Source: CAD feature listing. Evaluate the final solid. Frame: model axes, mm. Face numbers are marked on the shaded views. A direction names the side the tool comes from. Give positions to 0.01 mm unless a question says otherwise; leave off trailing zeros. Write each loop counter-clockwise with the first axis right and the second up, starting at its lowest first coordinate (ties: lowest second). Pieces come first, ordered by that corner, then holes. Notation, with made-up numbers: (-0.75, 52.25) -> (24.25, 52.25) arc R14 ccw to (24.25, 77.25) -> close; hole circle Ø9 at (63.5, -33). An arc over 180 degrees is marked (long way). Answer as a JSON object with one key per item and string values. Group by question number.
Item 1: Section query B-B on y = 16. Return the cut outline in (x, z) (1 decimal), plus the area to 3 significant figures.
Item 2: Section query A-A on z = -2125.5. Return the cut outline in (x, y), plus the area to 3 significant figures.
Item 3: Section query C-C on x = -18.5. Return the cut outline in (y, z), plus the area to 3 significant figures.
Item 4: Section query D-D on y = 61. Return the cut outline in (x, z), plus the area to 3 significant figures.
Item 5: Access query for the marked faces 4 and 5. Directions: +Z, -Z, +X, -X, +Y, -Y. A direction counts if a zero-diameter tool reaches every point of the face in a straight line with its end or side. Return the directions, or none.
Item 6: Pull-direction query (X, two-part tool) for the marked faces 1, 2 and 3; classes: pulls with the +X half, pulls with the -X half, needs draft (parallel to the pull), parting line crosses it, or undercut.
Item 7: Ray query, probe 1 along X at (y, z) = (5, -2128); probe 2 along Z at (x, y) = (28.5, 9); probe 3 along X at (y, z) = (24, -2125.25). Return the intervals inside material, ascending. Write a range as from..to.
Item 8: First-contact query: pin 1 Ø4.5 at (x, z) = (-39, -2123.5) entering from -Y; pin 2 Ø1.7 at (x, z) = (-25.5, -2116) entering from +Y; pin 3 Ø1.7 at (y, z) = (-16, -2116) entering from +X; pin 4 Ø8 at (y, z) = (61, -2123) entering from -X. Flat tips, straight axial feed; report the tip coordinate or a pass-through.
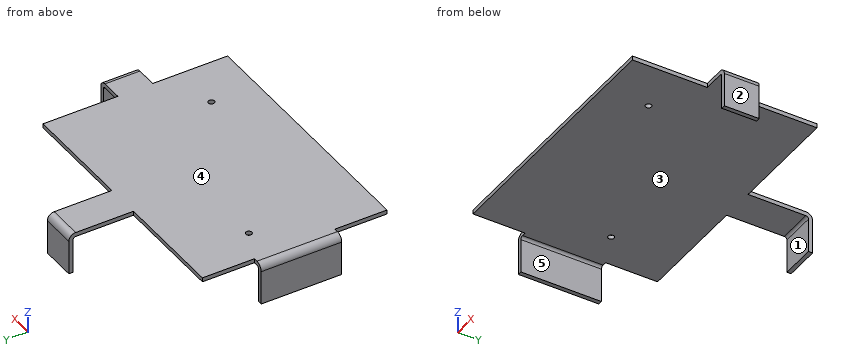
from build123d import *

# Parameters (mm, degrees)
BASE_FLANGE1_DEPTH             = 1.5875
EDGE_FLANGE1_STRIP_W           = 8.35
EDGE_FLANGE1_STRIP_H           = 1.5875
EDGE_FLANGE1_STRIP_CUT_DEPTH   = 30.48
EDGE_FLANGE1_STRIP_2_W         = 8.35
EDGE_FLANGE1_STRIP_2_H         = 1.5875
EDGE_FLANGE1_STRIP_CUT_2_DEPTH = 13.208
EDGE_FLANGE1_STRIP_3_W         = 8.35
EDGE_FLANGE1_STRIP_3_H         = 1.5875
EDGE_FLANGE1_STRIP_CUT_3_DEPTH = 13.208
EDGE_FLANGE1_DEPTH             = 30.48
EDGE_FLANGE1_BEND_DEPTH        = 13.208
EDGE_FLANGE1_BEND_2_DEPTH      = 13.208
F_4_40_TAPPED_HOLE2_D          = 2.2606
F_4_40_TAPPED_HOLE2_DEPTH      = 7.62
F_4_40_TAPPED_HOLE2_TIP        = 0.679152758


# Sheet-metal steps are written as plain solids
with BuildPart() as part:
    # Sketch4 → Base-Flange1 (new body)
    with BuildSketch(Plane.XY.offset(-2116.63312276)):
        Polygon((69.238438529, 17.87770801), (69.238438529, 4.66970801), (60.348438529, 4.66970801), (60.348438529, -23.65129199), (-37.441561471, -23.65129199), (-37.441561471, -3.96629199), (-39.981561471, -3.96629199), (-39.981561471, 26.51370801), (-37.441561471, 26.51370801), (-37.441561471, 46.19870801), (4.849438529, 46.19870801), (4.849438529, 69.05870801), (18.057438529, 69.05870801), (18.057438529, 46.19870801), (60.348438529, 46.19870801), (60.348438529, 17.87770801), align=None)
    extrude(amount=BASE_FLANGE1_DEPTH)

    # Edge-Flange1 strip (across the edge) → Edge-Flange1 strip cut (cut)
    with BuildSketch(Plane(origin=(-39.981561471, -3.96629199, -2116.63312276), x_dir=(1, 0, 0), z_dir=(0, 1, 0))):
        with Locations((-3.175, -0.79375)):
            Rectangle(EDGE_FLANGE1_STRIP_W, EDGE_FLANGE1_STRIP_H)
    extrude(amount=EDGE_FLANGE1_STRIP_CUT_DEPTH, mode=Mode.SUBTRACT)

    # Edge-Flange1 strip 2 (across the edge) → Edge-Flange1 strip cut 2 (cut)
    with BuildSketch(Plane(origin=(4.849438529, 69.05870801, -2116.63312276), x_dir=(0, -1, 0), z_dir=(1, 0, 0))):
        with Locations((-3.175, -0.79375)):
            Rectangle(EDGE_FLANGE1_STRIP_2_W, EDGE_FLANGE1_STRIP_2_H)
    extrude(amount=EDGE_FLANGE1_STRIP_CUT_2_DEPTH, mode=Mode.SUBTRACT)

    # Edge-Flange1 strip 3 (across the edge) → Edge-Flange1 strip cut 3 (cut)
    with BuildSketch(Plane(origin=(69.238438529, 17.87770801, -2116.63312276), x_dir=(-1, 0, 0), z_dir=(0, -1, 0))):
        with Locations((-3.175, -0.79375)):
            Rectangle(EDGE_FLANGE1_STRIP_3_W, EDGE_FLANGE1_STRIP_3_H)
    extrude(amount=EDGE_FLANGE1_STRIP_CUT_3_DEPTH, mode=Mode.SUBTRACT)

    # Edge-Flange1 section (across the edge) → Edge-Flange1 (add)
    with BuildSketch(Plane(origin=(-39.981561471, -3.96629199, -2116.63312276), x_dir=(1, 0, 0), z_dir=(0, 1, 0))):
        with BuildLine():
            Line((-1.5875, 1), (-1.5875, 13.97))
            Line((-1.5875, 13.97), (0, 13.97))
            Line((0, 13.97), (0, 1))
            ThreePointArc((0, 1), (0.292893219, 0.292893219), (1, 0))
            Line((1, 0), (1, -1.5875))
            ThreePointArc((1, -1.5875), (-0.829638796, -0.829638796), (-1.5875, 1))
        make_face()
    extrude(amount=EDGE_FLANGE1_DEPTH)

    # Edge-Flange1 section 2 (across the edge) → Edge-Flange1 bend (add)
    with BuildSketch(Plane(origin=(4.849438529, 69.05870801, -2116.63312276), x_dir=(0, -1, 0), z_dir=(1, 0, 0))):
        with BuildLine():
            Line((-1.5875, 1), (-1.5875, 13.97))
            Line((-1.5875, 13.97), (0, 13.97))
            Line((0, 13.97), (0, 1))
            ThreePointArc((0, 1), (0.292893219, 0.292893219), (1, 0))
            Line((1, 0), (1, -1.5875))
            ThreePointArc((1, -1.5875), (-0.829638796, -0.829638796), (-1.5875, 1))
        make_face()
    extrude(amount=EDGE_FLANGE1_BEND_DEPTH)

    # Edge-Flange1 section 3 (across the edge) → Edge-Flange1 bend 2 (add)
    with BuildSketch(Plane(origin=(69.238438529, 17.87770801, -2116.63312276), x_dir=(-1, 0, 0), z_dir=(0, -1, 0))):
        with BuildLine():
            Line((-1.5875, 1), (-1.5875, 13.97))
            Line((-1.5875, 13.97), (0, 13.97))
            Line((0, 13.97), (0, 1))
            ThreePointArc((0, 1), (0.292893219, 0.292893219), (1, 0))
            Line((1, 0), (1, -1.5875))
            ThreePointArc((1, -1.5875), (-0.829638796, -0.829638796), (-1.5875, 1))
        make_face()
    extrude(amount=EDGE_FLANGE1_BEND_2_DEPTH)

    # #4-40 Tapped Hole2
    with Locations(Plane(origin=(41.933438529, -6.18879199, -2115.04562276), x_dir=(1, 0, 0), z_dir=(0, 0, 1))):
        with Locations((0, 0), (-66.675, 26.9875)):
            Hole(F_4_40_TAPPED_HOLE2_D / 2, depth=F_4_40_TAPPED_HOLE2_DEPTH)
            with Locations((0, 0, -(F_4_40_TAPPED_HOLE2_DEPTH + F_4_40_TAPPED_HOLE2_TIP / 2))):  # 118° drill point
                Cone(0, F_4_40_TAPPED_HOLE2_D / 2, F_4_40_TAPPED_HOLE2_TIP, mode=Mode.SUBTRACT)


solid = part.part
Worked answers:
{
 "1": {"outline": "(-41.6, -2130.6) -> (-40, -2130.6) -> (-40, -2117.6) arc R1 cw to (-39, -2116.6) -> (68.2, -2116.6) arc R1 cw to (69.2, -2117.6) -> (69.2, -2130.6) -> (70.8, -2130.6) -> (70.8, -2117.6) arc R2.6 ccw to (68.2, -2115) -> (-39, -2115) arc R2.6 ccw to (-41.6, -2117.6) -> close", "area": "220 mm^2"},
 "2": {"outline": "(-41.57, -3.97) -> (-39.98, -3.97) -> (-39.98, 26.51) -> (-41.57, 26.51) -> close; (4.85, 69.06) -> (18.06, 69.06) -> (18.06, 70.65) -> (4.85, 70.65) -> close; (69.24, 4.67) -> (70.83, 4.67) -> (70.83, 17.88) -> (69.24, 17.88) -> close", "area": "90.3 mm^2"},
 "3": {"outline": "(-23.65, -2116.63) -> (46.2, -2116.63) -> (46.2, -2115.05) -> (-23.65, -2115.05) -> close", "area": "111 mm^2"},
 "4": {"outline": "(4.85, -2116.63) -> (18.06, -2116.63) -> (18.06, -2115.05) -> (4.85, -2115.05) -> close", "area": "21.0 mm^2"},
 "5": {"face 4": "+Z, +X, -X, +Y, -Y", "face 5": "-Z, +Y, -Y"},
 "6": {"face 1": "needs draft", "face 2": "pulls with the +X half", "face 3": "undercut"},
 "7": {"probe 1": "-41.57..-39.98, 69.24..70.83", "probe 2": "-2116.63..-2115.05", "probe 3": "-41.57..-39.98"},
 "8": {"pin 1": "y = -3.97", "pin 2": "y = 46.2", "pin 3": "x = 60.35", "pin 4": "through"}
}
